Autodesk Inventor part; units mm, degrees
ref_plane "YZ Plane" through (0, 0, 0) normal (1, 0, 0) x (0, 1, 0)
ref_plane "XZ Plane" through (0, 0, 0) normal (0, 1, 0) x (-1, 0, 0)
ref_plane "XY Plane" through (0, 0, 0) normal (0, 0, 1) x (1, 0, 0)
sketch "Sketch1" plane through (0, 0, 0) normal (0, 0, 1) x (1, 0, 0)
  arc A0 (-16.5011, 13.8506) -> (-21.6973, 4.8506) centre (-16.5011, 7.8506) ccw
  line L0 (-16.5011, 13.8506) -> (16.5011, 13.8506)
  arc A1 (21.6973, 4.8506) -> (16.5011, 13.8506) centre (16.5011, 7.8506) ccw
  line L1 (21.6973, 4.8506) -> (13.3257, -9.6494)
  arc A2 (5.5315, -14.1494) -> (13.3257, -9.6494) centre (5.5315, -5.1494) ccw
  line L2 (5.5315, -14.1494) -> (-5.5315, -14.1494)
  arc A3 (-13.3257, -9.6494) -> (-5.5315, -14.1494) centre (-5.5315, -5.1494) ccw
  line L3 (-13.3257, -9.6494) -> (-21.6973, 4.8506)
  line L4 (10, -20.5494) -> (10, -40.5494)
  line L5 (10, -40.5494) -> (-10, -40.5494)
  line L6 (-10, -40.5494) -> (-10, -20.5494)
  line L7 (-10, -20.5494) -> (10, -20.5494)
  line L8 (-43, 31.7481) -> (-15, -16.7494)
  line L9 (-15, -16.7494) -> (-32.2735, -26.7222)
  arc A4 (-32.2735, -26.7222) -> (32.2735, -26.7222) centre (0, -5.7301) ccw
  line L10 (32.2735, -26.7222) -> (15, -16.7494)
  line L11 (15, -16.7494) -> (43, 31.7481)
  line L12 (43, 31.7481) -> (38.6699, 34.2481)
  line L13 (38.6699, 34.2481) -> (31.7143, 22.2006)
  arc A5 (23.4871, 17.4506) -> (31.7143, 22.2006) centre (23.4871, 26.9506) ccw
  line L14 (23.4871, 17.4506) -> (-23.4871, 17.4506)
  arc A6 (-31.7143, 22.2006) -> (-23.4871, 17.4506) centre (-23.4871, 26.9506) ccw
  line L15 (-31.7143, 22.2006) -> (-38.6699, 34.2481)
  line L16 (-38.6699, 34.2481) -> (-43, 31.7481)
  arc A7 (-222.7491, 428.2441) -> (-227.9453, 437.2441) centre (-227.9453, 431.2441) ccw
  line L17 (-222.7491, 428.2441) -> (-239.2502, 399.6633)
  arc A8 (-249.6425, 399.6633) -> (-239.2502, 399.6633) centre (-244.4464, 402.6633) ccw
  line L18 (-249.6425, 399.6633) -> (-258.0141, 414.1633)
  arc A9 (-258.0141, 423.1633) -> (-258.0141, 414.1633) centre (-250.2199, 418.6633) ccw
  line L19 (-258.0141, 423.1633) -> (-252.4827, 432.7441)
  arc A10 (-244.6884, 437.2441) -> (-252.4827, 432.7441) centre (-244.6884, 428.2441) ccw
  line L20 (-244.6884, 437.2441) -> (-227.9453, 437.2441)
  line L21 (-265.791, 422.4934) -> (-283.1115, 432.4934)
  line L22 (-283.1115, 432.4934) -> (-273.1115, 449.8139)
  line L23 (-273.1115, 449.8139) -> (-255.791, 439.8139)
  line L24 (-255.791, 439.8139) -> (-265.791, 422.4934)
  line L25 (-194.0001, 442.2441) -> (-250.0001, 442.2441)
  line L26 (-250.0001, 442.2441) -> (-250.0001, 462.1898)
  arc A11 (-250.0001, 462.1898) -> (-282.2736, 406.2904) centre (-247.9571, 423.7441) ccw
  line L27 (-282.2736, 406.2904) -> (-265.0001, 416.2633)
  line L28 (-265.0001, 416.2633) -> (-237.0001, 367.7659)
  line L29 (-237.0001, 367.7659) -> (-232.6699, 370.2659)
  line L30 (-232.6699, 370.2659) -> (-239.6255, 382.3133)
  arc A12 (-239.6255, 391.8133) -> (-239.6255, 382.3133) centre (-231.3983, 387.0633) ccw
  line L31 (-239.6255, 391.8133) -> (-216.1385, 432.4941)
  arc A13 (-207.9112, 437.2441) -> (-216.1385, 432.4941) centre (-207.9112, 427.7441) ccw
  line L32 (-207.9112, 437.2441) -> (-194.0001, 437.2441)
  line L33 (-194.0001, 437.2441) -> (-194.0001, 442.2441)
  arc A14 (239.2501, 399.6635) -> (249.6424, 399.6635) centre (244.4463, 402.6635) ccw
  line L34 (239.2501, 399.6635) -> (222.749, 428.2443)
  arc A15 (227.9452, 437.2443) -> (222.749, 428.2443) centre (227.9452, 431.2443) ccw
  line L35 (227.9452, 437.2443) -> (244.6883, 437.2443)
  arc A16 (252.4825, 432.7443) -> (244.6883, 437.2443) centre (244.6883, 428.2443) ccw
  line L36 (252.4825, 432.7443) -> (258.014, 423.1635)
  arc A17 (258.014, 414.1635) -> (258.014, 423.1635) centre (250.2198, 418.6635) ccw
  line L37 (258.014, 414.1635) -> (249.6424, 399.6635)
  line L38 (255.7908, 439.8142) -> (273.1113, 449.8142)
  line L39 (273.1113, 449.8142) -> (283.1113, 432.4937)
  line L40 (283.1113, 432.4937) -> (265.7908, 422.4937)
  line L41 (265.7908, 422.4937) -> (255.7908, 439.8142)
  line L42 (237, 367.7661) -> (264.9999, 416.2635)
  line L43 (264.9999, 416.2635) -> (282.2735, 406.2907)
  arc A18 (282.2735, 406.2907) -> (249.9999, 462.19) centre (247.957, 423.7443) ccw
  line L44 (249.9999, 462.19) -> (249.9999, 442.2443)
  line L45 (249.9999, 442.2443) -> (193.9999, 442.2443)
  line L46 (193.9999, 442.2443) -> (193.9999, 437.2443)
  line L47 (193.9999, 437.2443) -> (207.9111, 437.2443)
  arc A19 (216.1383, 432.4943) -> (207.9111, 437.2443) centre (207.9111, 427.7443) ccw
  line L48 (216.1383, 432.4943) -> (239.6254, 391.8135)
  arc A20 (239.6254, 382.3135) -> (239.6254, 391.8135) centre (231.3982, 387.0635) ccw
  line L49 (239.6254, 382.3135) -> (232.6699, 370.2661)
  line L50 (232.6699, 370.2661) -> (237, 367.7661)
  line L51 (-194.0001, 442.2441) -> (193.9999, 442.2443)
  line L52 (193.9999, 442.2443) -> (237, 367.7661)
  line L53 (237, 367.7661) -> (43, 31.7481)
  line L54 (43, 31.7481) -> (-43, 31.7481)
  line L55 (-43, 31.7481) -> (-237.0001, 367.7659)
  line L56 (-237.0001, 367.7659) -> (-194.0001, 442.2441)
  line L57 (-247.9571, 423.7441) -> (0, 280.5861)
  line L58 (247.957, 423.7443) -> (0, 280.5861)
  line L59 (0, -5.7301) -> (0, 280.5861)
  line L60 (0, 280.5861) -> (140, 199.7571)
  line L61 (0, 280.5861) -> (-140, 199.757)
  line L62 (0, 280.5861) -> (-0.0001, 442.2442)
  point P0 (0, 0)
extrude "Extrusion1" add sketch "Sketch1" along normal blind 1.5 contours L61 L55 L29 L30 L56 L57 | L57 L56 L32 L33 L51 L62 | L30 L29 L56 | L56 L33 L32
properties part number "alu plate" material "Glass"
The listing builds one solid part. Answer for the finished solid, in the listing's coordinates (mm). Give positions to 0.01 mm unless a question says otherwise; leave off trailing zeros. Loops run counter-clockwise (first coordinate to the right, second up) from the corner with the lowest first, then second, coordinate; pieces in that order, holes last. Notation, with made-up numbers: (-9, -19.5) - (34, -19.5) arc R16 ccw to (34, -0.5) - close; hole circle Ø2 at (-39.75, -29). An arc over 180 degrees is marked (long way). Write each question's results on one line, items separated by ' | '.
1. Find section B-B, the plane x = -53.5. Write down the section's boundary in (y, z).
Resolved:
outline: (249.7, 0) - (442.24, 0) - (442.24, 1.5) - (249.7, 1.5) - close
2. Find section C-C, the plane y = 228. Write down the section's boundary in (x, z), then the cut area to 3 significant figures.
Resolved:
outline: (-156.31, 0) - (-91.08, 0) - (-91.08, 1.5) - (-156.31, 1.5) - close | area: 97.8 mm^2
3. Consider probe 1 along X at (y, z) = (431.5, 0.35); probe 2 along X at (y, z) = (360, 1.25); probe 3 along Y at (x, z) = (-80, 0.3). Determine where each line is inside the solid, lowest interval first. Write a range as from..to.
Resolved:
probe 1: x = -200.2..0 | probe 2: x = -232.52..0 | probe 3: y = 234.4..442.24
4. Find section A-A, the plane z = 0.45. Write down the section's boundary in (x, y), then the cut area to 3 significant figures.
Resolved:
outline: (-237, 367.77) - (-140, 199.76) - (0, 280.59) - (0, 442.24) - (-194, 442.24) - close | area: 42,100 mm^2
